from build123d import *

# Parameters (mm, degrees)
SKETCH_1_R          = 16.75
EXTRUDE_1_DEPTH     = 3
SKETCH_2_R          = 1.6
CUT_EXTRUDE_1_DEPTH = 3
SKETCH_3_R          = 6.6
CUT_EXTRUDE_2_DEPTH = 3
SKETCH_4_R          = 1.4
CUT_EXTRUDE_3_DEPTH = 10


with BuildPart() as part:
    # 草图1 → 凸台-拉伸1 (new body)
    with BuildSketch(Plane(origin=(0, 0, 0), x_dir=(1, 0, 0), z_dir=(0, 1, 0))):
        with Locations(Location((0, 0, 0), (0, 0, 270))):
            Circle(SKETCH_1_R)
    extrude(amount=EXTRUDE_1_DEPTH)

    # 草图2 → 切除-拉伸1 (cut)
    with BuildSketch(Plane(origin=(0, 3, 0), x_dir=(1, 0, 0), z_dir=(0, 1, 0))):
        with Locations(Location((4.75, 8.227241336, 0), (0, 0, 270))):
            Circle(SKETCH_2_R)
        with Locations(Location((4.75, -8.227241336, 0), (0, 0, 270))):
            Circle(SKETCH_2_R)
        with Locations(Location((-9.5, 0, 0), (0, 0, 270))):
            Circle(SKETCH_2_R)
    extrude(amount=-CUT_EXTRUDE_1_DEPTH, mode=Mode.SUBTRACT)

    # 草图3 → 切除-拉伸2 (cut)
    with BuildSketch(Plane(origin=(0, 3, 0), x_dir=(1, 0, 0), z_dir=(0, 1, 0))):
        with Locations(Location((0, 0, 0), (0, 0, 270))):
            Circle(SKETCH_3_R)
    extrude(amount=-CUT_EXTRUDE_2_DEPTH, mode=Mode.SUBTRACT)

    # 草图4 → 切除-拉伸3 (cut)
    with BuildSketch(Plane(origin=(0, 3, 0), x_dir=(1, 0, 0), z_dir=(0, 1, 0))):
        with Locations(Location((-14.75, 0, 0), (0, 0, 270))):
            Circle(SKETCH_4_R)
        with Locations(Location((7.375, 12.773874706, 0), (0, 0, 270))):
            Circle(SKETCH_4_R)
        with Locations(Location((7.375, -12.773874706, 0), (0, 0, 270))):
            Circle(SKETCH_4_R)
    extrude(amount=-CUT_EXTRUDE_3_DEPTH, mode=Mode.SUBTRACT)


solid = part.part
Verification items for the finished model (mm, model axes). Coordinates: 2 decimals unless noted, no trailing zeros. Write each loop counter-clockwise with the first axis right and the second up, starting at its lowest first coordinate (ties: lowest second). Pieces come first, ordered by that corner, then holes. Notation, with made-up numbers: (63.25, 12) -> (67.25, 12) arc R25 cw to (67.25, 45) -> close; hole circle Ø4 at (74.25, -15.5). An arc over 180 degrees is marked (long way). One line per item, written item: value. Start each with the question number.
Q1. Cross-section at D-D on z = 5.5. Enter the section's corners in (x, y), and give its area (3 significant figures).
Q2. Go/stop test with a flat-tipped pin: P1, Ø1, axis at y = 1, z = 2.5, coming from the +X side. Record where the tip stops, or that it passes through.
Q3. Cross-section at B-B on x = 0. Enter the section's corners in (y, z).
Q4. Mould release check, pull along X, two halves, no side actions. Record for faces 1 (the cylindrical face through (3.19, 1.52, 7.88)), 2 (the flat face through (0, 3, 7)), 3 (the cylindrical face through (-14.86, 1.48, 7.73)): pulls with the +X half, pulls with the -X half, needs draft (parallel to the pull), parting line crosses it, or undercut.
Q5. Cross-section at C-C on x = 8. Enter the section's corners in (y, z), and give its area (3 significant figures).
Q6. Thickness scan on L1, parallel to Z at x = 5, y = 1.05; L2, parallel to X at y = 1.4, z = 0; L3, parallel to Z at x = 8, y = 1. Record the ranges inside material, lowest first. Write a range as from..to.
Q7. Cross-section at A-A on z = 0. Enter the section's corners in (x, y).
Checked values:
1. outline: (-15.82, 0) -> (-3.65, 0) -> (-3.65, 3) -> (-15.82, 3) -> close; (3.65, 0) -> (15.82, 0) -> (15.82, 3) -> (3.65, 3) -> close
1. area: 73.0 mm²
2. P1: stops at x = 16.63
3. outline: (0, -16.75) -> (3, -16.75) -> (3, -6.6) -> (0, -6.6) -> close; (0, 6.6) -> (3, 6.6) -> (3, 16.75) -> (0, 16.75) -> close
4. face 1: undercut
4. face 2: needs draft
4. face 3: parting line crosses it
5. outline: (0, -14.72) -> (3, -14.72) -> (3, -14.03) -> (0, -14.03) -> close; (0, -11.52) -> (3, -11.52) -> (3, 11.52) -> (0, 11.52) -> close; (0, 14.03) -> (3, 14.03) -> (3, 14.72) -> (0, 14.72) -> close
5. area: 73.3 mm²
6. L1: z = -15.99..-9.81, -6.65..-4.31, 4.31..6.65, 9.81..15.99
6. L2: x = -16.75..-16.15, -13.35..-11.1, -7.9..-6.6, 6.6..16.75
6. L3: z = -14.72..-14.03, -11.52..11.52, 14.03..14.72
7. outline: (-16.75, 0) -> (-16.15, 0) -> (-16.15, 3) -> (-16.75, 3) -> close; (-13.35, 0) -> (-11.1, 0) -> (-11.1, 3) -> (-13.35, 3) -> close; (-7.9, 0) -> (-6.6, 0) -> (-6.6, 3) -> (-7.9, 3) -> close; (6.6, 0) -> (16.75, 0) -> (16.75, 3) -> (6.6, 3) -> close
